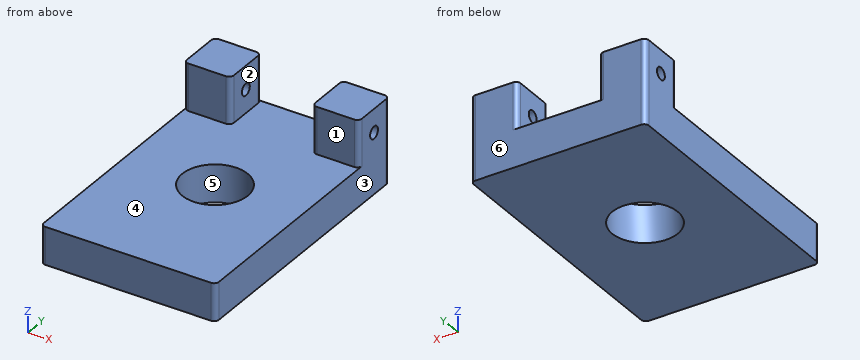
Autodesk Fusion 360 part; units mm, degrees
sketch "Sketch1" plane through (0, 0, 0) normal (0, 0, 1) x (1, 0, 0)
  line L0 (0.5, 0) -> (18.2, 0)
  line L1 (18.7, 0.5) -> (18.7, 28.2)
  line L2 (18.2, 28.7) -> (0.5, 28.7)
  line L3 (0, 28.2) -> (0, 0.5)
  line L4 (18.7, 28.7) -> (0, 0) construction
  line L5 (0, 28.7) -> (18.7, 0) construction
  arc A0 (0.5, 28.7) -> (0, 28.2) centre (0.5, 28.2) ccw
  arc A1 (18.7, 28.2) -> (18.2, 28.7) centre (18.2, 28.2) ccw
  arc A2 (18.2, 0) -> (18.7, 0.5) centre (18.2, 0.5) ccw
  arc A3 (0, 0.5) -> (0.5, 0) centre (0.5, 0.5) ccw
  circle A4 centre (9.35, 14.35) radius 3.5
  dimension "d1" = 18.7
  dimension "d2" = 28.7
  dimension "d3" = 0.5
  dimension "d4" = 0.5
  dimension "d5" = 0.5
  dimension "d6" = 0.5
  dimension "d7" = 7
extrude "Extrude1" add sketch "Sketch1" along normal blind 4
sketch "Sketch2" plane through (0, 0, 4) normal (0, 0, 1) x (-1, 0, 0)
  circle A0 centre (-9.35, -14.35) radius 3.5
  arc A1 (0, -0.5) -> (-0.5, 0) centre (-0.5, -0.5) ccw
  line L0 (-0.5, 0) -> (-18.2, 0)
  arc A2 (-18.2, 0) -> (-18.7, -0.5) centre (-18.2, -0.5) ccw
  line L1 (-18.7, -0.5) -> (-18.7, -28.2)
  arc A3 (-18.7, -28.2) -> (-18.2, -28.7) centre (-18.2, -28.2) ccw
  line L2 (-18.2, -28.7) -> (-0.5, -28.7)
  arc A4 (-0.5, -28.7) -> (0, -28.2) centre (-0.5, -28.2) ccw
  line L3 (0, -28.2) -> (0, -0.5)
  line L4 (-9.35, -23.7) -> (-18.2, -23.7) construction
  line L5 (-9.35, -23.7) -> (0, -23.7) construction
  line L6 (-18.7, -23.7) -> (-14.2, -23.7)
  line L7 (-0.5, -23.7) -> (-4.5, -23.7)
  line L8 (-5, -24.2) -> (-5, -28.2)
  line L9 (-13.7, -24.2) -> (-13.7, -28.2)
  line L10 (-14.2, -28.7) -> (-18.2, -28.7)
  line L11 (-18.7, -28.2) -> (-18.7, -24.2)
  line L12 (-4.5, -28.7) -> (-0.5, -28.7)
  line L13 (0, -28.2) -> (0, -24.2)
  arc A5 (-0.5, -28.7) -> (0, -28.2) centre (-0.5, -28.2) ccw
  arc A6 (-18.7, -28.2) -> (-18.2, -28.7) centre (-18.2, -28.2) ccw
  arc A7 (-4.5, -23.7) -> (-5, -24.2) centre (-4.5, -24.2) ccw
  arc A8 (0, -24.2) -> (-0.5, -23.7) centre (-0.5, -24.2) ccw
  arc A9 (-5, -28.2) -> (-4.5, -28.7) centre (-4.5, -28.2) ccw
  arc A10 (-14.2, -28.7) -> (-13.7, -28.2) centre (-14.2, -28.2) ccw
  arc A11 (-13.7, -24.2) -> (-14.2, -23.7) centre (-14.2, -24.2) ccw
  arc A12 (-18.2, -23.7) -> (-18.7, -24.2) centre (-18.2, -24.2) ccw
  point P0 (-5, -28.7)
  point P1 (-13.7, -28.7)
  point P2 (-18.7, -28.7)
  point P3 (0, -28.7)
  dimension "d12" = 5
  dimension "d13" = 5
  dimension "d14" = 0.5
  dimension "d15" = 0.5
  dimension "d16" = 0.5
  dimension "d17" = 0.5
  dimension "d18" = 0.5
  dimension "d19" = 0.5
  dimension "d20" = 0.5
  dimension "d21" = 0.5
extrude "Extrude2" add sketch "Sketch2" along normal blind 5 contours L2 A4 L3 L7 L8 L12 L13 A5 A7 A8 A9 | L1 A3 L2 L6 L9 L10 L11 A6 A10 A11 A12
sketch "Sketch3" plane through (18.7, 0, 0) normal (1, 0, 0) x (0, 1, 0)
  line L0 (0.5, 0) -> (28.2, 0)
  line L1 (28.2, 0) -> (28.2, 9)
  line L2 (28.2, 9) -> (24.2, 9)
  line L3 (24.2, 9) -> (24.2, 4)
  line L4 (24.2, 4) -> (0.5, 4)
  line L5 (0.5, 4) -> (0.5, 0)
  line L6 (24.2, 9) -> (24.2, 4) construction
  line L7 (24.2, 4) -> (28.2, 4) construction
  line L8 (24.2, 9) -> (28.2, 4) construction
  line L9 (24.2, 4) -> (28.2, 9) construction
  circle A0 centre (26.2, 6.5) radius 0.65
  dimension "d24" = 1.3
extrude "Extrude3" cut sketch "Sketch3" against normal blind 20 contours A0
The listing builds one solid part. Answer for the finished solid, in the listing's coordinates (mm). Face numbers are marked on the shaded views. A direction names the side the tool comes from. Round coordinates to 2 decimals unless told otherwise and drop trailing zeros. Order: outer loops, then holes, each group sorted by start corner. A loop starts at its lowest first (then second) coordinate and runs counter-clockwise, first axis right, second up. Notation, with made-up numbers: (9.25, 45.5) -> (43.25, 45.5) arc R23 cw to (43.25, 66.5) -> close; hole circle Ø5 at (13, 6). An arc over 180 degrees is marked (long way). Answer as CSV lines item,"result".
Q1. A cutting plane is placed at B-B on y = 26.2. Determine the outline of the cut face in (x, z).
Computed values:
outline,"(0, 0) -> (18.7, 0) -> (18.7, 5.85) -> (13.7, 5.85) -> (13.7, 4) -> (5, 4) -> (5, 5.85) -> (0, 5.85) -> close; (0, 7.15) -> (5, 7.15) -> (5, 9) -> (0, 9) -> close; (13.7, 7.15) -> (18.7, 7.15) -> (18.7, 9) -> (13.7, 9) -> close"
Q2. For a pull along Y with two mould halves and no side action, classify the marked faces 4, 5 and 6 as +Y half, -Y half, draft (parallel to the pull), parting line (faces both ways), or undercut.
Computed values:
face 4,"draft"
face 5,"undercut"
face 6,"+Y half"
Q3. Which of the six approach directions +Z, -Z, +X, -X, +Y, -Y give full straight-line access (tool end or side, diameter ignored) to the marked faces 1, 2 and 3?
Computed values:
face 1,"+Z, +X, -X, -Y"
face 2,"+Z, +Y, -Y"
face 3,"+Z, -Z, +X, +Y, -Y"
Q4. Given pin 1 (6 mm diameter, centred on x = 11, y = 5, fed in from +Z); pin 2 (2 mm diameter, centred on x = 3, z = 6, fed in from -Y), each flat-ended and moving along its own axis, determine where each tip first touches the part or whether it passes through.
Computed values:
pin 1,"stops at z = 4"
pin 2,"stops at y = 23.7"
Q5. A cutting plane is placed at A-A on z = 7.5. Determine the outline of the cut face in (x, y), plus the area to 3 significant figures.
Computed values:
outline,"(0, 24.2) arc R0.5 ccw to (0.5, 23.7) -> (4.5, 23.7) arc R0.5 ccw to (5, 24.2) -> (5, 28.2) arc R0.5 ccw to (4.5, 28.7) -> (0.5, 28.7) arc R0.5 ccw to (0, 28.2) -> close; (13.7, 24.2) arc R0.5 ccw to (14.2, 23.7) -> (18.2, 23.7) arc R0.5 ccw to (18.7, 24.2) -> (18.7, 28.2) arc R0.5 ccw to (18.2, 28.7) -> (14.2, 28.7) arc R0.5 ccw to (13.7, 28.2) -> close"
area,"49.6 mm^2"
Q6. Consider line 1 (Y direction, x = 9.35, z = 2.5); line 2 (Z direction, x = 17.5, y = 26.2); line 3 (Z direction, x = 10.75, y = 8.75). Determine where each line is inside the solid, lowest interval first. Write a range as from..to.
Computed values:
line 1,"y = 0..10.85, 17.85..28.7"
line 2,"z = 0..5.85, 7.15..9"
line 3,"z = 0..4"
Q7. A cutting plane is placed at D-D on x = 15. Determine the outline of the cut face in (y, z).
Computed values:
outline,"(0, 0) -> (28.7, 0) -> (28.7, 9) -> (23.7, 9) -> (23.7, 4) -> (0, 4) -> close; hole circle Ø1.3 at (26.2, 6.5)"
Q8. A cutting plane is placed at C-C on y = 12.25. Determine the outline of the cut face in (x, z), plus the area to 3 significant figures.
Computed values:
outline,"(0, 0) -> (6.55, 0) -> (6.55, 4) -> (0, 4) -> close; (12.15, 0) -> (18.7, 0) -> (18.7, 4) -> (12.15, 4) -> close"
area,"52.4 mm^2"
